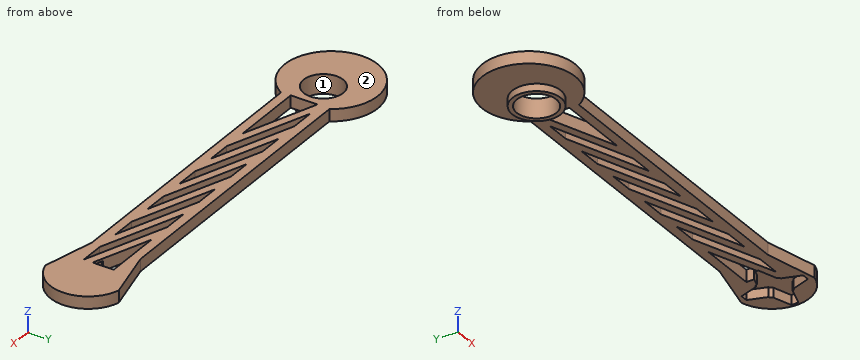
Autodesk Inventor part; units mm, degrees
ref_plane "Płaszczyzna konstrukcyjna1" through (-138.5, 0, -1) normal (0, 0, 1) x (1, 0, 0)
ref_plane "YZ Plane" through (0, 0, 0) normal (1, 0, 0) x (0, 1, 0)
ref_plane "XZ Plane" through (0, 0, 0) normal (0, 1, 0) x (-1, 0, 0)
sketch "Szkic1" plane through (0, 0, 0) normal (0, 1, 0) x (-1, 0, 0)
  line L0 (0, 0) -> (150, 0)
  line L1 (150, 0) -> (150, -5)
  line L2 (150, -5) -> (0, -5)
  line L3 (0, -5) -> (0, 0)
  dimension "d0" = 150
  dimension "d1" = 5
extrude "Wyciągnięcie proste1" add sketch "Szkic1" along normal blind 20
sketch "Szkic2" plane through (0, 0, -5) normal (0, 0, -1) x (-1, 0, 0)
  line L0 (0, 0) -> (0, 20)
  circle A0 centre (0, 10) radius 2.95
  line L1 (0, 20) -> (-2, 20)
  line L2 (0, 0) -> (-2, 0)
  arc A1 (-2, 20) -> (-2, 0) centre (9.1803, 10) ccw
  line L3 (0, 10) -> (150, 10)
  line L4 (150, 10) -> (138.5, 10)
  line L5 (138.5, 10) -> (170.9, 10)
  line L6 (150, 0) -> (150, 20)
  line L7 (138.5, 10) -> (170.9, 10) construction
  line L8 (138.5, 10) -> (170.9, 10)
  line L9 (170.9, 10) -> (170.9, 16.16)
  line L10 (170.9, 16.16) -> (138.5, 16.16)
  line L11 (138.5, 16.16) -> (138.5, 10)
  line L12 (138.5, 10) -> (170.9, 10)
  line L13 (170.9, 10) -> (170.9, 3.84)
  line L14 (170.9, 3.84) -> (138.5, 3.84)
  line L15 (138.5, 3.84) -> (138.5, 10)
  line L16 (0, 0) -> (150, 0)
  line L17 (0, 20) -> (150, 20)
  arc A2 (138.5, 0) -> (138.5, 20) centre (154.9429, 10) ccw
  point P0 (150, 3.84)
  point P1 (150, 16.16)
  point P2 (0, 7.05)
  point P3 (0, 12.95)
  dimension "d4" = 5.9
  dimension "d5" = 2
  dimension "d6" = 2
  dimension "d7" = 15
  dimension "d8" = 150
  dimension "d9" = 11.5
  dimension "d10" = 32.4
  dimension "d11" = 0
  dimension "d12" = 6.16
  dimension "d13" = 6.16
extrude "Wyciągnięcie proste2" add sketch "Szkic2" against normal blind 5 contours L2 A1 L1 L0 A0 | L16 L6 L14 L13 L9 L10 L17 A2
sketch "Szkic3" plane through (2, 20, -5) normal (0, 0, -1) x (-1, 0, 0)
  arc A0 (2, -7.05) -> (2, -12.95) centre (2, -10) ccw
  circle A1 centre (2, -10) radius 2.95
  line L0 (152, -16.16) -> (152, -3.84)
  line L1 (152, -16.16) -> (150.5, -16.16)
  line L2 (150.5, -16.16) -> (150.5, -3.84)
  line L3 (150.5, -3.84) -> (152, -3.84)
  line L4 (140.5, -16.16) -> (10.5, -16.16)
  line L5 (10.5, -16.16) -> (10.5, -3.84)
  line L6 (10.5, -3.84) -> (140.5, -3.84)
  line L7 (140.5, -3.84) -> (140.5, -16.16)
  line L8 (150.5, -16.16) -> (150.3, -16.16)
  line L9 (150.3, -16.16) -> (150.3, -3.84)
  line L10 (150.3, -3.84) -> (150.5, -3.84)
  line L11 (152, -16.16) -> (140.5, -16.16)
  line L12 (140.5, -16.16) -> (140.5, -3.84)
  line L13 (140.5, -3.84) -> (152, -3.84)
  line L14 (152, -3.84) -> (152, -16.16)
  point P0 (2, -20)
  dimension "d16" = 1.5
  dimension "d17" = 130
  dimension "d18" = 12.32
  dimension "d21" = 0.2
  dimension "d24" = 11.5
extrude "Wyciągnięcie proste3" cut sketch "Szkic3" against normal through all
sketch "Szkic5" plane through (2, 20, -5) normal (0, 0, -1) x (-1, 0, 0)
  circle A0 centre (2, -10) radius 2.95
  line L0 (2, -10) -> (152, -10)
  line L1 (2, -10) -> (152, -10) construction
  circle A1 centre (152, -10) radius 5.0551
  line L2 (152, -10) -> (145.8, -10)
  line L3 (145.8, -10) -> (145.8, -3.84)
  line L4 (10.5, -3.84) -> (172.9, -3.84)
  line L5 (145.8, -3.84) -> (140.8, -3.84)
  line L6 (140.8, -3.84) -> (140.8, -16.16)
  line L7 (172.9, -16.16) -> (10.5, -16.16)
  line L8 (145.8, -10) -> (145.8, -16.16)
  line L9 (145.8, -16.16) -> (140.8, -16.16)
  line L10 (10.5, -16.16) -> (10.5, -3.84)
  line L11 (10.5, -16.16) -> (44.3489, -3.84)
  line L12 (10.5, -16.16) -> (46.5213, -16.16) construction
  line L13 (44.3489, -3.84) -> (54.3489, -3.84)
  line L14 (10.5, -16.16) -> (20.5, -16.16)
  line L15 (20.5, -16.16) -> (54.3489, -3.84)
  line L16 (20.5, -16.16) -> (30.5, -16.16)
  line L17 (54.3489, -3.84) -> (64.3489, -3.84)
  line L18 (64.3489, -3.84) -> (30.5, -16.16)
  line L19 (44.3489, -3.84) -> (34.3489, -3.84)
  line L20 (10.5, -16.16) -> (0.5, -16.16)
  line L21 (0.5, -16.16) -> (34.3489, -3.84)
  line L22 (40.5, -16.16) -> (74.3489, -3.84)
  line L23 (50.5, -16.16) -> (84.3489, -3.84)
  line L24 (94.3489, -3.84) -> (60.5, -16.16)
  line L25 (30.5, -16.16) -> (64.3489, -3.84)
  line L26 (70.5, -16.16) -> (104.3489, -3.84)
  line L27 (80.5, -16.16) -> (114.3489, -3.84)
  line L28 (124.3489, -3.84) -> (90.5, -16.16)
  line L29 (60.5, -16.16) -> (94.3489, -3.84)
  line L30 (100.5, -16.16) -> (134.3489, -3.84)
  line L31 (110.5, -16.16) -> (144.3489, -3.84)
  line L32 (90.5, -16.16) -> (124.3489, -3.84)
  point P0 (2, -20)
  point P1 (10.5, -12.5203)
  point P2 (60.5, -16.16)
  point P3 (140.8, -5.1317)
  dimension "d25" = 150
  dimension "d26" = 0
  dimension "d27" = 6.2
  dimension "d28" = 5
  dimension "d29" = 20
  dimension "d30" = 10
  dimension "d31" = 10
  dimension "d32" = 10
  dimension "d33" = 10
  dimension "d34" = 10
  dimension "d35" = 10
  dimension "d36" = 10
  dimension "d37" = 10
  dimension "d38" = 10
  dimension "d39" = 10
  dimension "d40" = 10
  dimension "d41" = 10
  dimension "d42" = 10
  dimension "d43" = 10
  dimension "d44" = 10
  dimension "d45" = 10
  dimension "d46" = 10
  dimension "d47" = 10
  dimension "d48" = 10
  dimension "d49" = 10
  dimension "d52" = 10
  dimension "d53" = 10
extrude "Wyciągnięcie proste4" add sketch "Szkic5" against normal blind 5 contours L21 L4 L11 L0 | L0 L11 L10 L21 | L15 L4 L18 L0 | L0 L18 L7 L15 | L22 L4 L23 L0 | L0 L23 L7 L22 | L24 L4 L26 L0 | L0 L26 L7 L24 | L27 L4 L28 L0 | L0 L28 L7 L27 | L30 L4 L6 L31 L0 | L0 L31 L7 L30 | L6 L31 L4 L3 L0 | L0 L8 L7 L6 | L6 L4 L31
sketch "Szkic6" plane through (-138.5, 0, 0) normal (0, 0, 1) x (1, 0, 0)
  circle A0 centre (138.5, 10) radius 2.95
  circle A1 centre (138.5, 10) radius 2.85
  circle A2 centre (138.5, 10) radius 2.95
  point P0 (138.5, 0)
  dimension "d56" = 5.7
extrude "Wyciągnięcie proste5" add sketch "Szkic6" against normal blind 5
ref_plane "Płaszczyzna konstrukcyjna1" through (-138.5, 0, -1) normal (0, 0, 1) x (1, 0, 0)
sketch "Szkic7" plane through (-138.5, 0, -1) normal (0, 0, 1) x (1, 0, 0)
  circle A0 centre (138.5, 10) radius 2.85
  circle A1 centre (138.5, 10) radius 1.25
  circle A2 centre (138.5, 10) radius 2.85
  point P0 (138.5, 0)
  dimension "d60" = 2.5
extrude "Wyciągnięcie proste6" add sketch "Szkic7" against normal blind 1
sketch "Szkic8" plane through (-138.5, 0, 0) normal (0, 0, 1) x (1, 0, 0)
  point P0 (138.5, 0)
sketch "Szkic9" plane through (-138.5, 0, 0) normal (0, 0, 1) x (1, 0, 0)
  circle A0 centre (138.5, 10) radius 1.25
  line L0 (138.5, 10) -> (-11.5, 10)
  line L1 (138.5, 10) -> (288.5, 10) construction
  circle A1 centre (-11.5, 10) radius 8.15
  point P0 (138.5, 0)
  dimension "d63" = 150
  dimension "d64" = 180
  dimension "d65" = 16.3
extrude "Wyciągnięcie proste7" cut sketch "Szkic9" against normal through all contours A1
sketch "Szkic10" plane through (-138.5, 0, 0) normal (0, 0, 1) x (1, 0, 0)
  arc A0 (-5.3, 4.7102) -> (-5.3, 15.2898) centre (-11.5, 10) ccw
  circle A1 centre (-11.5, 10) radius 8.15
  line L0 (-32.5164, 20) -> (-2.9538, 20)
  line L1 (-2.9538, 20) -> (-2.9538, 1.85)
  line L2 (-2.9538, 1.85) -> (-32.5164, 1.85)
  line L3 (-32.5164, 1.85) -> (-32.5164, 20)
  point P0 (138.5, 0)
  point P1 (-11.5, 1.85)
  point P2 (-5.3, 15.2898)
extrude "Wyciągnięcie proste8" add sketch "Szkic10" against normal blind 5
sketch "Szkic11" plane through (2, 20, -5) normal (0, 0, -1) x (-1, 0, 0)
  circle A0 centre (152, -10) radius 8.15
  circle A1 centre (152, -10) radius 8.15
  circle A2 centre (152, -10) radius 10
  point P0 (2, -20)
  dimension "d70" = 20
extrude "Wyciągnięcie proste9" add sketch "Szkic11" along normal blind 3
sketch "Szkic12" plane through (2, 20, -5) normal (0, 0, -1) x (-1, 0, 0)
  circle A0 centre (2, -10) radius 1.25
  circle A1 centre (2, -10) radius 5.2
  arc A2 (0, 0) -> (0, -20) centre (11.1803, -10) ccw
  line L0 (2, -10) -> (14.7, -10)
  line L1 (2, -10) -> (2, 2.7)
  line L2 (2, -10) -> (-10.7, -10)
  line L3 (2, -10) -> (2, -22.7)
  line L4 (2, -15.2) -> (6, -15.2)
  line L5 (6, -15.2) -> (2, -15.2)
  line L6 (2, -15.2) -> (-2, -15.2)
  line L7 (7.2, -10) -> (7.2, -6)
  line L8 (7.2, -10) -> (7.2, -14)
  line L9 (2, -4.8) -> (-2, -4.8)
  line L10 (2, -4.8) -> (6, -4.8)
  line L11 (-3.2, -10) -> (-3.2, -14)
  line L12 (-3.2, -10) -> (-3.2, -6)
  line L13 (2, -22.7) -> (3.5, -22.7)
  line L14 (3.5, -22.7) -> (2, -22.7)
  line L15 (2, -22.7) -> (0.5, -22.7)
  line L16 (3.5, -22.7) -> (6, -15.2)
  line L17 (0.5, -22.7) -> (-2, -15.2)
  line L18 (14.7, -8.5) -> (7.2, -6)
  line L19 (14.7, -11.5) -> (7.2, -14)
  line L20 (14.7, -8.5) -> (14.7, -10)
  line L21 (0.5, 2.7) -> (-2, -4.8)
  line L22 (3.5, 2.7) -> (6, -4.8)
  line L23 (0.5, 2.7) -> (2, 2.7)
  line L24 (-10.7, -11.5) -> (-3.2, -14)
  line L25 (-10.7, -8.5) -> (-3.2, -6)
  line L26 (-10.7, -11.5) -> (-10.7, -10)
  line L27 (-10.7, -11.5) -> (-10.7, -8.5)
  line L28 (14.7, -11.5) -> (14.7, -8.5)
  line L29 (3.5, 2.7) -> (0.5, 2.7)
  arc A3 (7.2, -6) -> (6, -4.8) centre (5.3194, -6.6806) ccw
  arc A4 (-2, -4.8) -> (-3.2, -6) centre (-1.3194, -6.6806) ccw
  arc A5 (-3.2, -14) -> (-2, -15.2) centre (-1.3194, -13.3194) ccw
  arc A6 (6, -15.2) -> (7.2, -14) centre (5.3194, -13.3194) ccw
  point P0 (2, -20)
  dimension "d73" = 10.4
  dimension "d75" = 12.7
  dimension "d76" = 12.7
  dimension "d77" = 12.7
  dimension "d78" = 12.7
  dimension "d79" = 4
  dimension "d80" = 4
  dimension "d83" = 360
  dimension "d85" = 1.5
  dimension "d86" = 1.5
  dimension "d89" = 360
  dimension "d91" = 2
  dimension "d92" = 2
  dimension "d93" = 2
  dimension "d94" = 2
sketch "Szkic13" plane through (2, 20, -5) normal (0, 0, -1) x (-1, 0, 0)
  line L0 (140.5, 0) -> (0, 0)
  line L1 (21.4996, 0) -> (0, 5.1324)
  arc A0 (0, 0) -> (0, -20) centre (11.1803, -10) ccw
  line L2 (-3.8197, -10) -> (24.797, -10)
  line L3 (21.4996, -20) -> (0, -25.1324)
  arc A1 (0, 5.1324) -> (0, -25.1324) centre (3.8411, -10) ccw
  line L4 (21.4996, 0) -> (21.4996, -20)
  line L5 (140.5, -20) -> (0, -20)
  point P0 (2, -20)
extrude "Wyciągnięcie proste10" add sketch "Szkic13" against normal blind 5 contours L0 A0 L5 L3 A1 L1
extrude "Wyciągnięcie proste11" cut sketch "Szkic12" against normal blind 4 contours L0 L1 A0 | L0 A1 L3 A0 | A0 L3 L0 | A0 L1 A1 L0 | L1 L2 A0 | A0 L2 A1 L1 | L3 A1 L2 A0 | A0 L2 L3 | L8 A6 L4 A1 | L7 L18 L20 L0 | A1 L10 A3 L7 | L0 L28 L19 L8 | L9 L21 L23 L1 | A1 L12 A4 L9 | L1 L29 L22 L10 | L6 A5 L11 A1 | L4 L16 L13 L3 | L3 L15 L17 L6 | L11 L24 A2 L2 | L2 A2 L25 L12 | L2 L27 L25 A2 | A2 L24 L26 L2
ref_plane "Płaszczyzna konstrukcyjna2" through (-22.3, 8.5, -5) normal (-1, 0, 0) x (0, 0, 1)
sketch "Szkic14" plane through (-154.9429, 10, 0) normal (0, 0, 1) x (1, 0, 0)
  circle A0 centre (154.9429, 0) radius 2.85
  circle A1 centre (154.9429, 0) radius 2.85
  point P0 (154.9429, -10)
extrude "Wyciągnięcie proste12" add sketch "Szkic14" against normal blind 1
properties part number "arm_v3"
Model file for the job. Use its own axes, mm. Face numbers are marked on the shaded views. Give positions to 0.01 mm unless a question says otherwise; leave off trailing zeros. Loops run counter-clockwise (first coordinate to the right, second up) from the corner with the lowest first, then second, coordinate; pieces in that order, holes last. Notation, with made-up numbers: (-19.75, 61) - (-8.75, 61) arc R15 ccw to (-8.75, 69) - close; hole circle Ø10 at (3.5, 86.25). An arc over 180 degrees is marked (long way). One line per item, written item: value. Start each with the question number.
1. Probe L1, parallel to Y at x = -63, z = -3.75; L2, parallel to X at y = 10.5, z = -6.25; L3, parallel to Z at x = -59.5, y = 8. List the from-to ranges inside material, lowest first. Write a range as from..to.
2. Pin check, flat tips, straight feed: pin 1 (4 mm diameter, centred on x = -63.5, z = -3.5, fed in from +Y); pin 2 (3.5 mm diameter, centred on x = -0.5, z = -3, fed in from +Y); pin 3 (0.9 mm diameter, centred on x = 0.5, z = -4, fed in from -Y); pin 4 (1.5 mm diameter, centred on x = -133, z = -7, fed in from -Y). Stop position of each tip, or through.
3. Slice it at A-A (x = -147). List the corners of the cut face in (y, z), plus the area to 3 significant figures.
4. Pull direction Y, two halves, no side cores. Call the marked faces 1 and 2: pulls with the +Y half, pulls with the -Y half, needs draft (parallel to the pull), parting line crosses it, or undercut.
Solution:
1. L1: y = 0..5.48, 9.12..12.76, 16.16..20
1. L2: x = -159.99..-158.13, -141.87..-140.01
1. L3: z = -5..0
2. pin 1: stops at y = 20
2. pin 2: stops at y = 24.95
2. pin 3: stops at y = -4.88
2. pin 4: passes through
3. outline: (-7.53, -5) - (0.46, -5) - (0.46, -8) - (2.42, -8) - (2.42, 0) - (-7.53, 0) - close; (17.58, -8) - (19.54, -8) - (19.54, -5) - (27.53, -5) - (27.53, 0) - (17.58, 0) - close
3. area: 111 mm^2
4. face 1: undercut
4. face 2: needs draft
